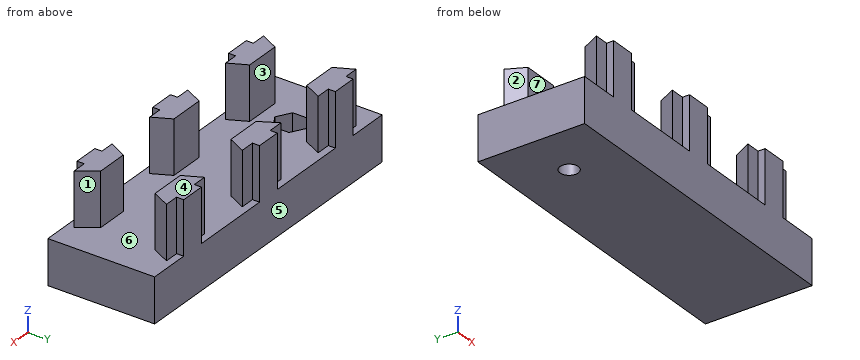
Autodesk Fusion 360 part; units mm, degrees
sketch "Sketch1" plane through (0, 0, 0) normal (0, 0, 1) x (1, 0, 0)
  line L0 (0, 0) -> (30, 0)
  line L1 (30, 0) -> (30, 30)
  line L2 (30, 30) -> (0, 30)
  line L3 (0, 30) -> (0, 0)
  dimension "d1" = 30
  dimension "d2" = 30
extrude "Extrude1" add sketch "Sketch1" along normal blind 12.5
sketch "Sketch2" plane through (0, 0, 12.5) normal (0, 0, 1) x (-1, 0, 0)
  line L0 (0, -30) -> (0, 0)
  line L1 (0, 0) -> (-30, 0)
  line L2 (-30, 0) -> (-30, -30)
  line L3 (-30, -30) -> (0, -30)
  line L4 (-15, -30) -> (-11.5, -30)
  line L5 (-15, -30) -> (-18.5, -30)
  line L6 (-18.5, -30) -> (-18.5, -28)
  line L7 (-11.5, -30) -> (-11.5, -28)
  line L8 (-15, -28) -> (-22.5, -28)
  line L9 (-15, -28) -> (-7.5, -28)
  line L10 (-15, -30) -> (-15, -23)
  line L11 (-15, -23) -> (-10, -23)
  line L12 (-15, -23) -> (-20, -23)
  line L13 (-10, -23) -> (-7.5, -28)
  line L14 (-20, -23) -> (-22.5, -28)
  dimension "d5" = 3.5
  dimension "d6" = 3.5
  dimension "d7" = 7.5
  dimension "d8" = 7.5
  dimension "d9" = 7
  dimension "d10" = 5
  dimension "d11" = 5
extrude "Extrude2" add sketch "Sketch2" along normal blind 15 contours L3 L4 L7 L9 L10 | L3 L5 L6 L8 L10 | L9 L10 L11 L13 | L8 L10 L12 L14
sketch "Sketch3" plane through (0, 0, 12.5) normal (0, 0, 1) x (-1, 0, 0)
  line L0 (-18.5, -30) -> (-18.5, -28)
  line L1 (-18.5, -28) -> (-22.5, -28)
  line L2 (-22.5, -28) -> (-20, -23)
  line L3 (-20, -23) -> (-10, -23)
  line L4 (-10, -23) -> (-7.5, -28)
  line L5 (-7.5, -28) -> (-11.5, -28)
  line L6 (-11.5, -28) -> (-11.5, -30)
  line L7 (-11.5, -30) -> (0, -30)
  line L8 (0, -30) -> (0, 0)
  line L9 (0, 0) -> (-30, 0)
  line L10 (-30, 0) -> (-30, -30)
  line L11 (-30, -30) -> (-18.5, -30)
  line L12 (-11.5, 0) -> (-11.5, -2)
  line L13 (-18.5, 0) -> (-18.5, -2)
  line L14 (-11.5, -2) -> (-7.5, -2)
  line L15 (-18.5, -2) -> (-22.5, -2)
  line L16 (-15, 0) -> (-15, -7)
  line L17 (-15, -7) -> (-20, -7)
  line L18 (-20, -7) -> (-22.5, -2)
  line L19 (-15, -7) -> (-10, -7)
  line L20 (-7.5, -2) -> (-10, -7)
  dimension "d15" = 4
  dimension "d16" = 4
  dimension "d17" = 7
  dimension "d18" = 5
extrude "Extrude3" add sketch "Sketch3" along normal blind 15 contours L9 L13 L15 L16 L17 L18 | L9 L12 L14 L16 L19 L20
sketch "Sketch4" plane through (0, 0, 12.5) normal (0, 0, 1) x (-1, 0, 0)
  line L0 (-18.5, -2) -> (-18.5, 0)
  line L1 (-18.5, 0) -> (-30, 0)
  line L2 (-30, 0) -> (-30, -30)
  line L3 (-30, -30) -> (-18.5, -30)
  line L4 (-18.5, -30) -> (-18.5, -28)
  line L5 (-18.5, -28) -> (-22.5, -28)
  line L6 (-22.5, -28) -> (-20, -23)
  line L7 (-20, -23) -> (-10, -23)
  line L8 (-10, -23) -> (-7.5, -28)
  line L9 (-7.5, -28) -> (-11.5, -28)
  line L10 (-11.5, -28) -> (-11.5, -30)
  line L11 (-11.5, -30) -> (0, -30)
  line L12 (0, -30) -> (0, 0)
  line L13 (0, 0) -> (-11.5, 0)
  line L14 (-11.5, 0) -> (-11.5, -2)
  line L15 (-11.5, -2) -> (-7.5, -2)
  line L16 (-7.5, -2) -> (-10, -7)
  line L17 (-10, -7) -> (-20, -7)
  line L18 (-20, -7) -> (-22.5, -2)
  line L19 (-22.5, -2) -> (-18.5, -2)
  line L20 (-15, -10.5) -> (-18.8971, -12.75)
  line L21 (-18.8971, -12.75) -> (-18.8971, -17.25)
  line L22 (-18.8971, -17.25) -> (-15, -19.5)
  line L23 (-15, -19.5) -> (-11.1029, -17.25)
  line L24 (-11.1029, -17.25) -> (-11.1029, -12.75)
  line L25 (-11.1029, -12.75) -> (-15, -10.5)
  point P0 (-15, -15)
  dimension "d21" = 4.5
extrude "Extrude4" cut sketch "Sketch4" against normal blind 6 contours L20 L21 L22 L23 L24 L25
sketch "Sketch5" plane through (0, 0, 6.5) normal (0, 0, 1) x (-1, 0, 0)
  line L0 (-11.1029, -12.75) -> (-15, -10.5)
  line L1 (-15, -10.5) -> (-18.8971, -12.75)
  line L2 (-18.8971, -12.75) -> (-18.8971, -17.25)
  line L3 (-18.8971, -17.25) -> (-15, -19.5)
  line L4 (-15, -19.5) -> (-11.1029, -17.25)
  line L5 (-11.1029, -17.25) -> (-11.1029, -12.75)
  circle A0 centre (-15, -15) radius 2.55
  dimension "d24" = 5.1
extrude "Extrude5" cut sketch "Sketch5" against normal blind 50 contours A0
sketch "Sketch6" plane through (0, 0, 0) normal (0, 0, 1) x (1, 0, 0)
  line L0 (30, 0) -> (90, 0)
  line L1 (90, 0) -> (90, 30)
  line L2 (90, 30) -> (30, 30)
  line L3 (30, 30) -> (30, 0)
  dimension "d27" = 60
extrude "Extrude6" add sketch "Sketch6" along normal blind 12.5
sketch "Sketch7" plane through (0, 0, 12.5) normal (0, 0, 1) x (-1, 0, 0)
  line L0 (-18.8971, -12.75) -> (-15, -10.5)
  line L1 (-15, -10.5) -> (-11.1029, -12.75)
  line L2 (-11.1029, -12.75) -> (-11.1029, -17.25)
  line L3 (-11.1029, -17.25) -> (-15, -19.5)
  line L4 (-15, -19.5) -> (-18.8971, -17.25)
  line L5 (-18.8971, -17.25) -> (-18.8971, -12.75)
  line L6 (-18.5, -2) -> (-18.5, 0)
  line L7 (-18.5, 0) -> (-90, 0)
  line L8 (-90, 0) -> (-90, -30)
  line L9 (-90, -30) -> (-18.5, -30)
  line L10 (-18.5, -30) -> (-18.5, -28)
  line L11 (-18.5, -28) -> (-22.5, -28)
  line L12 (-22.5, -28) -> (-20, -23)
  line L13 (-20, -23) -> (-10, -23)
  line L14 (-10, -23) -> (-7.5, -28)
  line L15 (-7.5, -28) -> (-11.5, -28)
  line L16 (-11.5, -28) -> (-11.5, -30)
  line L17 (-11.5, -30) -> (0, -30)
  line L18 (0, -30) -> (0, 0)
  line L19 (0, 0) -> (-11.5, 0)
  line L20 (-11.5, 0) -> (-11.5, -2)
  line L21 (-11.5, -2) -> (-7.5, -2)
  line L22 (-7.5, -2) -> (-10, -7)
  line L23 (-10, -7) -> (-20, -7)
  line L24 (-20, -7) -> (-22.5, -2)
  line L25 (-22.5, -2) -> (-18.5, -2)
  line L26 (0, -15) -> (-30, -15)
  line L27 (-90, -15) -> (-60, -15)
  line L28 (-41.5, 0) -> (-41.5, -2)
  line L29 (-48.5, 0) -> (-48.5, -2)
  line L30 (-48.5, -2) -> (-52.5, -2)
  line L31 (-41.5, -2) -> (-37.5, -2)
  line L32 (-45, -7) -> (-50, -7)
  line L33 (-50, -7) -> (-52.5, -2)
  line L34 (-45, -7) -> (-40, -7)
  line L35 (-40, -7) -> (-37.5, -2)
  line L36 (-45, -23) -> (-40, -23)
  line L37 (-45, -23) -> (-50, -23)
  line L38 (-41.5, -30) -> (-41.5, -28)
  line L39 (-48.5, -30) -> (-48.5, -28)
  line L40 (-48.5, -28) -> (-52.5, -28)
  line L41 (-41.5, -28) -> (-41.2186, -28)
  line L42 (-41.2186, -28) -> (-37.2186, -28)
  line L43 (-37.2186, -28) -> (-40, -23)
  line L44 (-50, -23) -> (-52.5, -28)
  line L45 (-75, -23) -> (-70, -23)
  line L46 (-70, -23) -> (-75, -23)
  line L47 (-75, -23) -> (-80, -23)
  line L48 (-71.5, -30) -> (-71.5, -28)
  line L49 (-78.5, -30) -> (-78.5, -28)
  line L50 (-71.5, -28) -> (-67.5, -28)
  line L51 (-70, -23) -> (-67.5, -28)
  line L52 (-80, -23) -> (-82.5, -28)
  line L53 (-82.5, -28) -> (-78.5, -28)
  line L54 (-71.413, 0) -> (-71.413, -2)
  line L55 (-78.413, 0) -> (-78.413, -2)
  line L56 (-78.413, -2) -> (-82.413, -2)
  line L57 (-71.413, -2) -> (-67.413, -2)
  line L58 (-75, -7) -> (-70, -7)
  line L59 (-70, -7) -> (-67.413, -2)
  line L60 (-75, -7) -> (-79, -7)
  line L61 (-79, -7) -> (-82.413, -2)
  dimension "d30" = 30
extrude "Extrude7" add sketch "Sketch7" along normal blind 15 contours L9 L36 L37 L38 L39 L40 L41 L42 L43 L44 | L7 L28 L29 L30 L31 L32 L33 L34 L35 | L9 L45 L46 L47 L48 L49 L50 L51 L52 L53 | L7 L54 L55 L56 L57 L58 L59 L60 L61
equation "d7 = ( 15 / 2 ) * 1 mm"
equation "d21 = ( 9 / 2 ) * 1 mm"
Work out the finished part from the listing and answer in its coordinate system (mm). Face numbers are marked on the shaded views. A direction names the side the tool comes from. Round coordinates to 2 decimals unless told otherwise and drop trailing zeros. Write each loop counter-clockwise with the first axis right and the second up, starting at its lowest first coordinate (ties: lowest second). Pieces come first, ordered by that corner, then holes.
1) A cutting plane is placed at C-C on x = 77.5. Determine the outline of the cut face in (y, z).
2) Consider probe 1 along X at (y, z) = (16.5, 8.25); probe 2 along Y at (x, z) = (15, 2.25); probe 3 along X at (y, z) = (15, 2). Determine where each line is inside the solid, lowest interval first.
3) Determine the mould class of the marked faces 4, 5, 6 and 7 for opening direction Y: pulls with the +Y half, pulls with the -Y half, needs draft (parallel to the pull), parting line crosses it, or undercut.
4) Which of the six approach directions +Z, -Z, +X, -X, +Y, -Y give full straight-line access (tool end or side, diameter ignored) to the marked faces 1, 2 and 3?
5) A cutting plane is placed at A-A on y = 15. Determine the outline of the cut face in (x, z).
6) A cutting plane is placed at B-B on z = 9. Determine the outline of the cut face in (x, y), and give its area (3 significant figures).
7) A cutting plane is placed at D-D on z = 25. Give the number of separate pieces and of enclosed holes in the cut face, and give its area (3 significant figures).
8) Flat-ended cylindrical pins translate along their axes: P1, Ø2, axis at x = 68.5, z = 17.5, coming from the +Y side; P2, Ø2, axis at x = 23, y = 19.5, coming from the +Z side; P3, Ø1, axis at x = 65, z = 22.5, coming from the -Y side; P4, Ø1.6, axis at y = 1, z = 19, coming from the +X side. Find the tip coordinate at first contact, or state that the pin passes through.
Entries:
1. outline: (0, 0) - (30, 0) - (30, 27.5) - (23, 27.5) - (23, 12.5) - (7, 12.5) - (7, 27.5) - (0, 27.5) - close
2. probe 1: x = 0 to 11.1, 18.9 to 90
2. probe 2: y = 0 to 12.45, 17.55 to 30
2. probe 3: x = 0 to 12.45, 17.55 to 90
3. face 4: needs draft
3. face 5: pulls with the +Y half
3. face 6: undercut
3. face 7: undercut
4. face 1: +Z, +X
4. face 2: +Z, -X
4. face 3: +Z, +X, -X
5. outline: (0, 0) - (12.45, 0) - (12.45, 6.5) - (11.1, 6.5) - (11.1, 12.5) - (0, 12.5) - close; (17.55, 0) - (90, 0) - (90, 12.5) - (18.9, 12.5) - (18.9, 6.5) - (17.55, 6.5) - close
6. outline: (0, 0) - (90, 0) - (90, 30) - (0, 30) - close; hole (11.1, 12.75) - (15, 10.5) - (18.9, 12.75) - (18.9, 17.25) - (15, 19.5) - (11.1, 17.25) - close
6. area: 2,650 mm2
7. separate pieces: 6
7. enclosed holes: 0
7. area: 457 mm2
8. P1: stops at y = 28
8. P2: stops at z = 12.5
8. P3: passes through
8. P4: stops at x = 78.41
